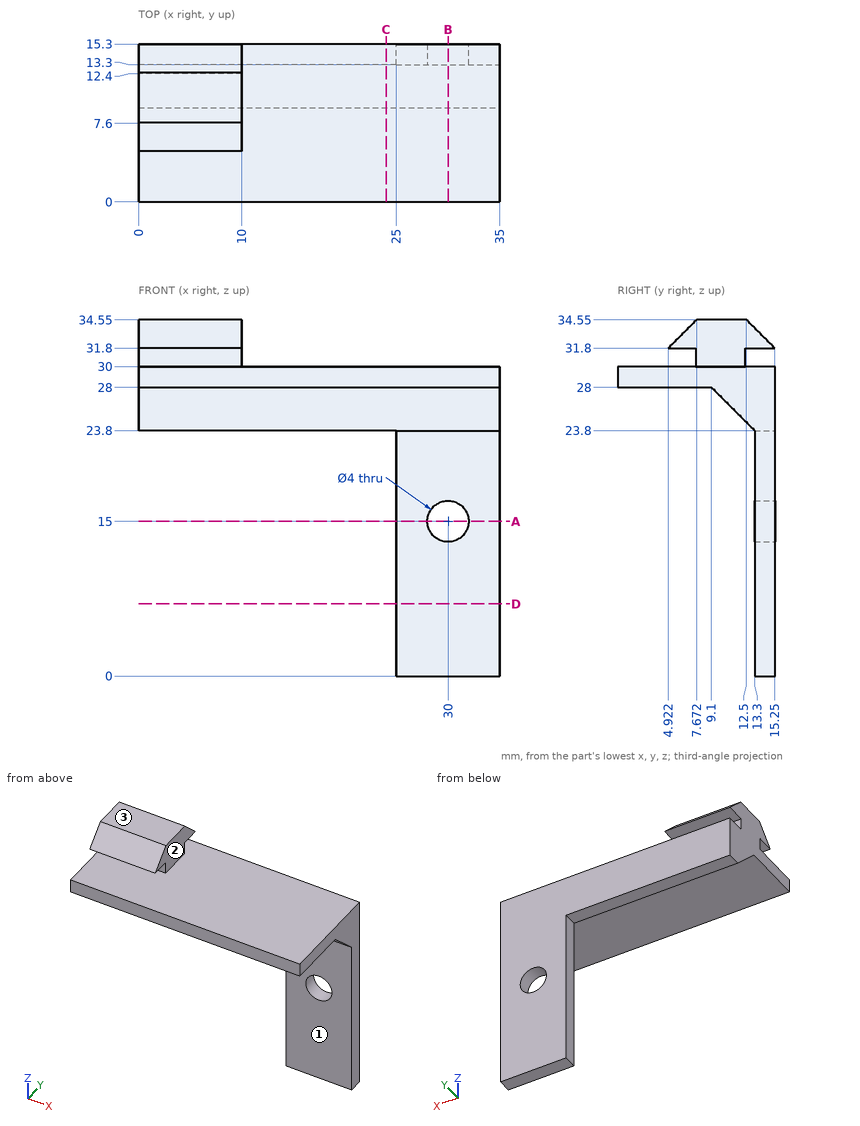
Here's the drawing with two shaded views (mm, measured from the low corner). I have some questions. A direction names the side the tool comes from. Coordinates: 2 decimals unless noted, no trailing zeros. Write each loop counter-clockwise with the first axis right and the second up, starting at its lowest first coordinate (ties: lowest second). Pieces come first, ordered by that corner, then holes. Notation, with made-up numbers: (71.25, -4) -> (115.25, -4) arc R19 ccw to (115.25, 16) -> close; hole circle Ø5 at (77.25, 9.25). An arc over 180 degrees is marked (long way). Write item = value, one per line. Start each with the question number.
(1) I want a section at A-A (z = 15). Please give me the cut outline in (x, y), plus the area to 3 significant figures.
(2) I need wall thicknesses on line 1 (Z direction, x = 30, y = 13.95); line 2 (Z direction, x = 11, y = 1.5); line 3 (Z direction, x = 12, y = 14.5). Which ranges of each line are inside material? Lowest first, please. Write a range as [from, to].
(3) Which directions (+Z, -Z, +X, -X, +Y, -Y) give clear straight access to the entire face, cutting with the end or side of a thin tool? Please do the marked faces 1, 2 and 3.
(4) I want a section at D-D (z = 7). Please give me the cut outline in (x, y), plus the area to 3 significant figures.
(5) I want a section at B-B (x = 30). Please give me the cut outline in (y, z).
(6) Will these pins go through, and if not, where does the flat tip stop? pin 1 (2 mm diameter, centred on x = 7, y = 14.5, fed in from -Z); pin 2 (5 mm diameter, centred on x = 28.5, y = 8, fed in from -Z); pin 3 (3 mm diameter, centred on x = 5, y = 6.5, fed in from -Z); pin 4 (2 mm diameter, centred on x = 7, z = 30.5, fed in from +Y).
(7) I want a section at C-C (x = 24). Please give me the cut outline in (y, z).
Result set:
q1.outline = (25, 13.3) -> (28, 13.3) -> (28, 15.3) -> (25, 15.3) -> close; (32, 13.3) -> (35, 13.3) -> (35, 15.3) -> (32, 15.3) -> close
q1.area = 12.0 mm2
q2.line_1 = [0, 13], [17, 30]
q2.line_2 = [28, 30]
q2.line_3 = [23.8, 30]
q3.face_1 = -Z, +X, -X, -Y
q3.face_2 = +Z, +X, +Y, -Y
q3.face_3 = +Z, +X, -X, +Y, -Y
q4.outline = (25, 13.3) -> (35, 13.3) -> (35, 15.3) -> (25, 15.3) -> close
q4.area = 20.0 mm2
q5.outline = (0, 28) -> (9.1, 28) -> (13.3, 23.8) -> (13.3, 17) -> (15.3, 17) -> (15.3, 30) -> (0, 30) -> close; (13.3, 0) -> (15.3, 0) -> (15.3, 13) -> (13.3, 13) -> close
q6.pin_1 = 23.8
q6.pin_2 = 26.6
q6.pin_3 = 28
q6.pin_4 = 15.3
q7.outline = (0, 28) -> (9.1, 28) -> (13.3, 23.8) -> (15.3, 23.8) -> (15.3, 30) -> (0, 30) -> close
